Geometry check sheet. Reference: the model listing, model coordinates, mm. Face numbers are marked on the shaded views. A direction names the side the tool comes from. Coordinates: 2 decimals unless noted, no trailing zeros. Order: outer loops, then holes, each group sorted by start corner. A loop starts at its lowest first (then second) coordinate and runs counter-clockwise, first axis right, second up.
```python
from build123d import *

# Parameters (mm, degrees)
CYLINDER003_R          = 2.5
CYLINDER003_DEPTH      = 22
CYLINDER002_R          = 10
CYLINDER002_DEPTH      = 10
LINEAREXTRUDE002_DEPTH = 10


with BuildPart() as cylinder003:
    # cylinder003 → cylinder003 (new body)
    with BuildSketch(Plane.XY.offset(-1)):
        Circle(CYLINDER003_R)
    extrude(amount=CYLINDER003_DEPTH)


with BuildPart() as cylinder002:
    # cylinder002 → cylinder002 (new body)
    with BuildSketch(Plane.XY.offset(10)):
        Circle(CYLINDER002_R)
    extrude(amount=CYLINDER002_DEPTH)


with BuildPart() as difference003:
    # union002 → LinearExtrude002 (new body)
    with BuildSketch(Plane(origin=(0, 0, 0), x_dir=(0, 1, 0), z_dir=(0, 0, 1))):
        Polygon((0.711931, -4.306123), (1.370771, -4.143733), (1.502069, -4.540636), (1.530367, -4.602072), (1.641751, -4.771632), (1.871155, -5.020002), (2.245545, -5.309618), (2.782207, -5.596589), (3.025427, -5.468937), (3.094113, -4.864255), (3.068442, -4.391617), (2.994354, -4.061731), (2.918082, -3.873743), (2.883597, -3.815555), (2.631538, -3.482032), (3.139447, -3.032064), (3.440155, -3.322487), (3.493763, -3.363735), (3.671187, -3.46211), (3.989737, -3.575421), (4.455834, -3.657875), (5.064387, -3.662577), (5.220426, -3.436516), (5.000234, -2.869177), (4.757857, -2.462607), (4.53895, -2.204938), (4.384052, -2.073928), (4.326475, -2.038431), (3.948292, -1.860249), (4.188912, -1.225786), (4.590143, -1.343197), (4.656779, -1.354807), (4.859597, -1.359461), (5.194318, -1.311756), (5.645345, -1.168159), (6.186377, -0.889514), (6.219486, -0.616832), (5.76086, -0.216806), (5.357304, 0.030555), (5.043726, 0.156979), (4.845688, 0.200998), (4.77821, 0.205671), (4.36054, 0.187693), (4.278749, 0.861305), (4.688584, 0.943805), (4.752983, 0.964491), (4.934732, 1.054624), (5.208943, 1.252418), (5.541575, 1.58917), (5.891142, 2.087328), (5.793738, 2.344162), (5.201743, 2.485233), (4.729457, 2.516719), (4.393046, 2.482935), (4.197235, 2.429879), (4.135314, 2.402658), (3.773841, 2.192639), (3.388376, 2.751081), (3.712928, 3.01459), (3.760337, 3.062835), (3.879381, 3.227107), (4.030263, 3.529677), (4.168298, 3.982437), (4.246318, 4.585986), (4.040715, 4.768136), (3.45097, 4.617935), (3.018149, 4.426332), (2.735972, 4.240079), (2.587247, 4.102103), (2.545069, 4.049224), (2.322601, 3.695276), (1.721767, 4.010618), (1.886685, 4.394771), (1.906243, 4.459522), (1.93531, 4.6603), (1.928298, 4.99833), (1.840114, 5.463378), (1.628715, 6.034052), (1.362012, 6.099788), (0.909622, 5.692724), (0.61542, 5.321926), (0.452121, 5.025874), (0.384552, 4.834585), (0.371779, 4.768162), (0.339281, 4.351371), (-0.339281, 4.351371), (-0.371779, 4.768162), (-0.384552, 4.834585), (-0.452121, 5.025874), (-0.61542, 5.321926), (-0.909622, 5.692724), (-1.362012, 6.099788), (-1.628715, 6.034052), (-1.840114, 5.463378), (-1.928298, 4.99833), (-1.93531, 4.6603), (-1.906243, 4.459522), (-1.886685, 4.394771), (-1.721767, 4.010618), (-2.322601, 3.695276), (-2.545069, 4.049224), (-2.587247, 4.102103), (-2.735972, 4.240079), (-3.018149, 4.426332), (-3.45097, 4.617935), (-4.040715, 4.768136), (-4.246318, 4.585986), (-4.168298, 3.982437), (-4.030263, 3.529677), (-3.879381, 3.227107), (-3.760337, 3.062835), (-3.712928, 3.01459), (-3.388376, 2.751081), (-3.773841, 2.192638), (-4.135314, 2.402658), (-4.197235, 2.429879), (-4.393046, 2.482935), (-4.729457, 2.516719), (-5.201743, 2.485233), (-5.793738, 2.344162), (-5.891142, 2.087328), (-5.541575, 1.58917), (-5.208943, 1.252418), (-4.934732, 1.054624), (-4.752983, 0.964491), (-4.688584, 0.943805), (-4.278749, 0.861305), (-4.36054, 0.187693), (-4.77821, 0.205671), (-4.845688, 0.200998), (-5.043726, 0.156979), (-5.357304, 0.030555), (-5.76086, -0.216806), (-6.219486, -0.616832), (-6.186377, -0.889514), (-5.645345, -1.168159), (-5.194318, -1.311756), (-4.859597, -1.359461), (-4.656779, -1.354807), (-4.590143, -1.343197), (-4.188912, -1.225786), (-3.948292, -1.860249), (-4.326475, -2.038431), (-4.384052, -2.073928), (-4.53895, -2.204938), (-4.757857, -2.462607), (-5.000234, -2.869177), (-5.220426, -3.436516), (-5.064387, -3.662577), (-4.455834, -3.657875), (-3.989737, -3.575421), (-3.671187, -3.46211), (-3.493763, -3.363735), (-3.440155, -3.322487), (-3.139447, -3.032064), (-2.631537, -3.482032), (-2.883597, -3.815555), (-2.918082, -3.873743), (-2.994354, -4.061731), (-3.068442, -4.391617), (-3.094113, -4.864255), (-3.025427, -5.468937), (-2.782207, -5.596589), (-2.245545, -5.309618), (-1.871155, -5.020002), (-1.641751, -4.771632), (-1.530367, -4.602072), (-1.502069, -4.540636), (-1.370771, -4.143733), (-0.71193, -4.306122), (-0.780122, -4.71858), (-0.783616, -4.78613), (-0.763789, -4.98803), (-0.676085, -5.31456), (-0.47917, -5.74499), (-0.137342, -6.24849), (0.137342, -6.24849), (0.47917, -5.74499), (0.676085, -5.31456), (0.763789, -4.98803), (0.783616, -4.78613), (0.780122, -4.71858), align=None)
    extrude(amount=LINEAREXTRUDE002_DEPTH)

    # union003: union cylinder002
    add(cylinder002.part)

    # difference003: cut cylinder003
    add(cylinder003.part, mode=Mode.SUBTRACT)


solid = difference003.part
```
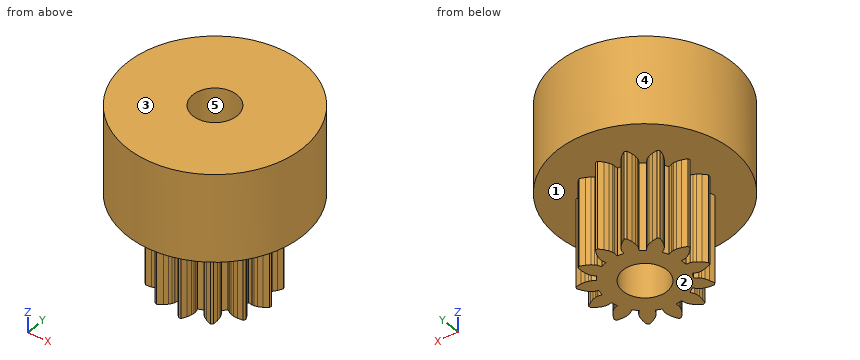
Item 1: Thickness scan on line 1 along Y through (x, z) = (0, 15.5); line 2 along X through (y, z) = (0, 6.5); line 3 along Z through (x, y) = (2, 6). Record the ranges inside material, lowest first.
Item 2: Tool access check on the marked faces 1 and 2. Record the directions out of +Z, -Z, +X, -X, +Y, -Y that give a thin tool (end or side, any length) a straight path to the whole face; none if there is none.
Item 3: Sectioned sample at A-A (y = 8). Record the cut outline in (x, z), and give its area (3 significant figures).
Item 4: Sectioned sample at B-B (z = 16). Record the cut outline in (x, y), and give its area (3 significant figures).
Item 5: Depth check by flat-ended pin: P1, Ø0.5, axis at y = 0, z = 7, coming from the -X side; P2, Ø8, axis at x = -5.5, z = 3.5, coming from the -Y side; P3, Ø4, axis at y = -5.5, z = 14, coming from the -X side. Enter the tip coordinate at first touch or a pass-through.
Item 6: Sectioned sample at C-C (x = 6.75). Record the cut outline in (y, z).
Item 7: Release check for a two-part mould opening along Y. For the marked faces 3, 4 and 5 record: pulls with the +Y half, pulls with the -Y half, needs draft (parallel to the pull), parting line crosses it, or undercut.
Geometry check:
1. line 1: y = -10 to -2.5, 2.5 to 10
1. line 2: x = -4.35 to -2.5, 2.5 to 6.25
1. line 3: z = 10 to 20
2. face 1: -Z
2. face 2: -Z, +X, -X, +Y, -Y
3. outline: (-6, 10) - (6, 10) - (6, 20) - (-6, 20) - close
3. area: 120 mm2
4. outline: circle Ø20 at (0, 0); hole circle Ø5 at (0, 0)
4. area: 295 mm2
5. P1: stops at x = -4.35
5. P2: stops at y = -5.89
5. P3: stops at x = -9.37
6. outline: (-7.38, 10) - (7.38, 10) - (7.38, 20) - (-7.38, 20) - close
7. face 3: needs draft
7. face 4: parting line crosses it
7. face 5: undercut
